```python
from build123d import *

# Parameters (mm, degrees)
BOX_W     = 40
BOX_H     = 40
BOX_DEPTH = 3
FILLET_R  = 3


with BuildPart() as con001:
    # Cone001 → Cone001 (revolve)
    with BuildSketch(Plane.XZ):
        Polygon((0, 0), (15, 0), (3, 40), (0, 40), align=None)
    revolve(axis=Axis((0, 0, 0), (0, 0, 1)))


with BuildPart() as cut:
    # Cone → Cone (revolve)
    with BuildSketch(Plane.XZ):
        Polygon((0, 0), (16, 0), (4, 40), (0, 40), align=None)
    revolve(axis=Axis((0, 0, 0), (0, 0, 1)))

    # Cut: cut Con001
    add(con001.part, mode=Mode.SUBTRACT)


with BuildPart() as cut_1:
    # Cut placement: moved
    add(cut.part.moved(Location((20, 20, 0))))


with BuildPart() as fusion:
    # Box → Box (new body)
    with BuildSketch(Plane.XY):
        with Locations((20, 20)):
            Rectangle(BOX_W, BOX_H)
    extrude(amount=BOX_DEPTH)

    # Fillet
    fillet_edges = [fusion.edges().sort_by_distance(p)[0] for p in [
        (0, 0, 1.5),
        (0, 40, 1.5),
        (40, 0, 1.5),
        (40, 40, 1.5),
    ]]
    fillet(fillet_edges, radius=FILLET_R)

    # Fusion: union Cut
    add(cut_1.part)


solid = fusion.part
```
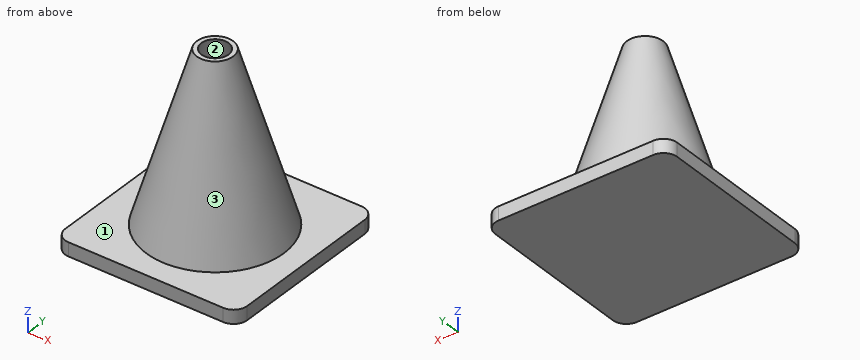
Check sheet for the modelled part. Datum: model origin and axes. Units: mm. Face numbers are marked on the shaded views. Round coordinates to 2 decimals unless told otherwise and drop trailing zeros. Loops run counter-clockwise (first coordinate to the right, second up) from the corner with the lowest first, then second, coordinate; pieces in that order, holes last. Notation, with made-up numbers: M -17.75,10.25 L 41.25,10.25 A30 cw 41.25,45.25 Z; hole C 85,76.5 d7. An arc over 180 degrees is marked long. Answer as a JSON object with one key per item and string values.
1. Section check C-C (z = 32). Record the boundary of the cut face in (x, y), plus the area to 3 significant figures.
Reply:
{"outline": "C 20,20 d12.8; hole C 20,20 d10.8", "area": "37.1 mm²"}
2. Section check D-D (z = 6). Record the boundary of the cut face in (x, y), plus the area to 3 significant figures.
Reply:
{"outline": "C 20,20 d28.4; hole C 20,20 d26.4", "area": "86.1 mm²"}
3. Mould release check, pull along X, two halves, no side actions. Record for the marked faces 1, 2 and 3: pulls with the +X half, pulls with the -X half, needs draft (parallel to the pull), parting line crosses it, or undercut.
Reply:
{"face 1": "needs draft", "face 2": "undercut", "face 3": "parting line crosses it"}
4. Scan lines: line 1 (X direction, y = 17.5, z = 21); line 2 (Y direction, x = 22, z = 18); line 3 (Y direction, x = 17.5, z = 32.5). Record each from-to range of solid material in increasing order.
Reply:
{"line 1": "x = 10.63 to 11.67, 28.33 to 29.37", "line 2": "y = 9.59 to 10.61, 29.39 to 30.41", "line 3": "y = 14.27 to 15.38, 24.62 to 25.73"}
5. Gauge pin test, flat ends, axial feed: P1, Ø1.5, axis at x = 20, z = 17.5, coming from the -Y side (3 decimals); P2, Ø2, axis at x = 29, z = 9, coming from the -Y side; P3, Ø10, axis at y = 16.5, z = 16.5, coming from the -X side. Record the tip position at first contact, or that the pin passes through.
Reply:
{"P1": "stops at y = 9.025", "P2": "stops at y = 9.29", "P3": "stops at x = 7.67"}
6. Section check A-A (y = 20). Record the boundary of the cut face in (x, z).
Reply:
{"outline": "M 0,0 L 40,0 L 40,3 L 35.1,3 L 24,40 L 23,40 L 34.1,3 L 5.9,3 L 17,40 L 16,40 L 4.9,3 L 0,3 Z"}
